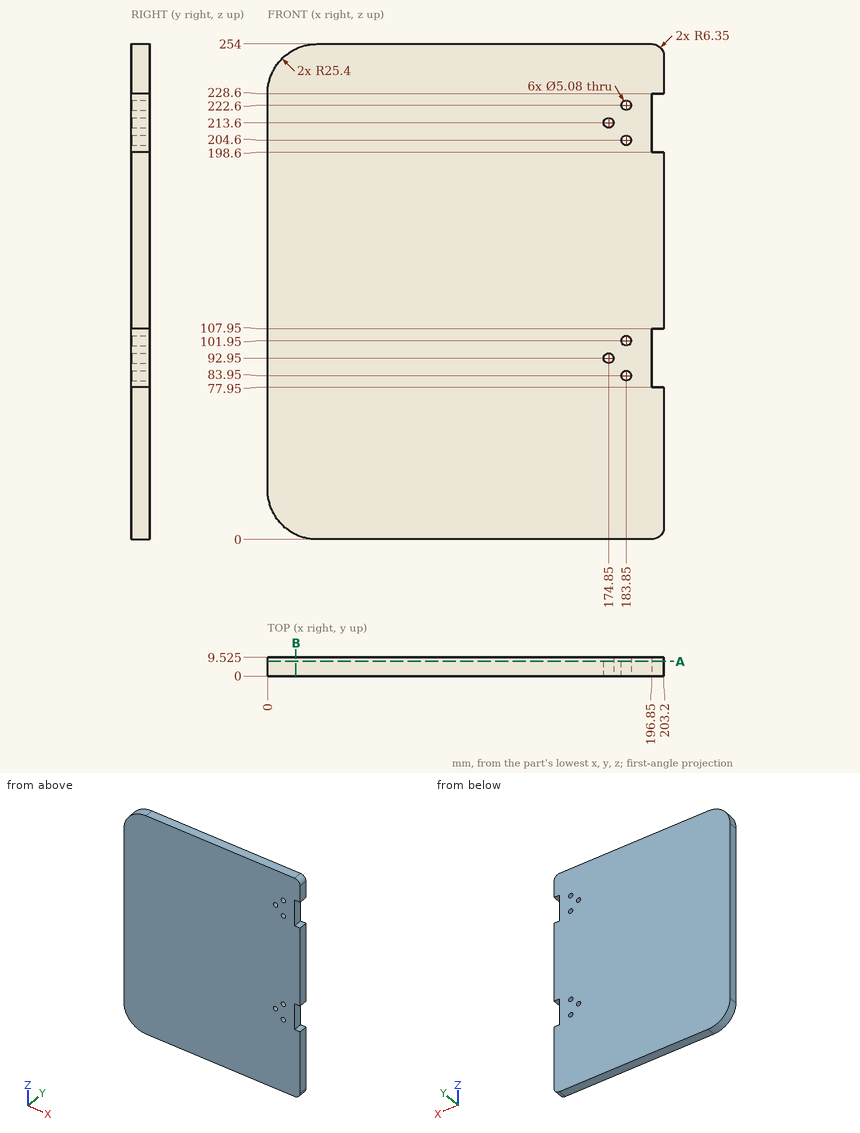
The figure shows three views and two pictorial views of one solid part (mm, origin at its lowest corner). Answer the questions. Give positions to 0.01 mm unless a question says otherwise; leave off trailing zeros. Loops run counter-clockwise (first coordinate to the right, second up) from the corner with the lowest first, then second, coordinate; pieces in that order, holes last. Notation, with made-up numbers: (-23.5, 13) -> (-5.5, 13) arc R21 ccw to (-5.5, 51) -> close; hole circle Ø11 at (-1.5, 68.5). An arc over 180 degrees is marked (long way). Use a Markdown table: item, result. Add a question column.
1. Section B-B on x = 14.5 is taken. Determine the outline of the cut face in (y, z) (3 decimals).
2. Section A-A on y = 7.5 is taken. Determine the outline of the cut face in (x, z), and give its area (3 significant figures).
3. Find the intervals of material crossed by probe 1 along Z at (x, y) = (183.85, 7); probe 2 along X at (y, z) = (1.5, 223); probe 3 along Z at (x, y) = (174.85, 3.5), in increasing order.
4. Flat-ended cylindrical pins translate along their axes: pin 1 Ø1.9 at (x, y) = (200.5, 4) entering from -Z; pin 2 Ø4 at (x, z) = (174.85, 213.6) entering from -Y; pin 3 Ø3 at (y, z) = (6, 215) entering from +X; pin 4 Ø1.9 at (x, y) = (200.5, 3) entering from +Z. Find the tip coordinate at first contact, or state that the pin passes through.
Results below:
| question | item | result |
|---|---|---|
| 1 | outline | (0, 2.458) -> (9.525, 2.458) -> (9.525, 251.542) -> (0, 251.542) -> close |
| 2 | outline | (0, 25.4) arc R25.4 ccw to (25.4, 0) -> (196.85, 0) arc R6.35 ccw to (203.2, 6.35) -> (203.2, 77.95) -> (196.85, 77.95) -> (196.85, 107.95) -> (203.2, 107.95) -> (203.2, 198.6) -> (196.85, 198.6) -> (196.85, 228.6) -> (203.2, 228.6) -> (203.2, 247.65) arc R6.35 ccw to (196.85, 254) -> (25.4, 254) arc R25.4 ccw to (0, 228.6) -> close; hole circle Ø5.08 at (174.85, 92.95); hole circle Ø5.08 at (174.85, 213.6); hole circle Ø5.08 at (183.85, 83.95); hole circle Ø5.08 at (183.85, 101.95); hole circle Ø5.08 at (183.85, 204.6); hole circle Ø5.08 at (183.85, 222.6) |
| 2 | area | 50,800 mm^2 |
| 3 | probe 1 | z = 0 to 81.41, 86.49 to 99.41, 104.49 to 202.06, 207.14 to 220.06, 225.14 to 254 |
| 3 | probe 2 | x = 0 to 181.34, 186.36 to 196.85 |
| 3 | probe 3 | z = 0 to 90.41, 95.49 to 211.06, 216.14 to 254 |
| 4 | pin 1 | stops at z = 0.6 |
| 4 | pin 2 | passes through |
| 4 | pin 3 | stops at x = 196.85 |
| 4 | pin 4 | stops at z = 253.4 |
